Work out the finished part from the listing and answer in its coordinate system (mm). A direction names the side the tool comes from. Coordinates: 2 decimals unless noted, no trailing zeros. Order: outer loops, then holes, each group sorted by start corner. A loop starts at its lowest first (then second) coordinate and runs counter-clockwise, first axis right, second up.
1. The part is cut by section D-D, the plane y = 23.5. Give the vertices of the cut face in (x, z).
2. The part is cut by section C-C, the plane z = 4.5. Give the vertices of the cut face in (x, y), then the cut area to 3 significant figures.
3. A tool of negligible diameter and unlimited length cuts with its end or side. For faces 4 (the flat face through (0, 2, 2)), 5 (the flat face through (18, 34, 3.5)), 6 (the flat face through (18, 33, 4)), from which of +Z, -Z, +X, -X, +Y, -Y can it reach the whole face along a straight path? Write none if from no direction.
4. A flat-ended cylindrical pin translates along its axis: pin 1 Ø1.5 at (y, z) = (17, 2) entering from -X. Find the tip coordinate at first contact, or state that the pin passes through.
5. Determine the mould class of faces 1 (the flat face through (20, 0, 2)), 2 (the flat face through (18, 5, 1)), 3 (the flat face through (20, 38, 2)) for opening direction Y: +Y half, -Y half, draft (parallel to the pull), parting line (faces both ways), or undercut.
6. The part is cut by section A-A, the plane x = 19. Give the vertices of the cut face in (y, z).
7. The part is cut by section B-B, the plane y = 34. Give the vertices of the cut face in (x, z).
8. Find the intervals of material crossed by probe 1 along Y at (x, z) = (2.5, 4.85); probe 2 along Y at (x, z) = (6.5, 2.65); probe 3 along Z at (x, y) = (31, 34), in increasing order.
```python
from build123d import *

# Parameters (mm, degrees)
ESQUISSE1_W             = 41
ESQUISSE1_H             = 38
BOSS_EXTRU_1_DEPTH      = 5
ESQUISSE6_W             = 36
ESQUISSE6_H             = 21
ENL_V_MAT_EXTRU_3_DEPTH = 5
ESQUISSE7_W             = 2
ESQUISSE7_H             = 32
ENL_V_MAT_EXTRU_4_DEPTH = 36
ESQUISSE8_W             = 5
ESQUISSE8_H             = 28
ENL_V_MAT_EXTRU_5_DEPTH = 36


with BuildPart() as part:
    # Esquisse1 → Boss.-Extru.1 (new body)
    with BuildSketch(Plane.XY):
        with Locations((20.5, 19)):
            Rectangle(ESQUISSE1_W, ESQUISSE1_H)
    extrude(amount=BOSS_EXTRU_1_DEPTH)

    # Esquisse6 → Enlèv. mat.-Extru.3 (cut)
    with BuildSketch(Plane(origin=(0, 0, 0), x_dir=(-1, 0, 0), z_dir=(0, 0, -1))):
        with Locations((-18, 19)):
            Rectangle(ESQUISSE6_W, ESQUISSE6_H)
    extrude(amount=-ENL_V_MAT_EXTRU_3_DEPTH, mode=Mode.SUBTRACT)

    # Esquisse7 → Enlèv. mat.-Extru.4 (cut)
    with BuildSketch(Plane.ZY):
        with Locations((2.5, 19)):
            Rectangle(ESQUISSE7_W, ESQUISSE7_H)
    extrude(amount=-ENL_V_MAT_EXTRU_4_DEPTH, mode=Mode.SUBTRACT)

    # Esquisse8 → Enlèv. mat.-Extru.5 (cut)
    with BuildSketch(Plane.ZY):
        with Locations((2.5, 19)):
            Rectangle(ESQUISSE8_W, ESQUISSE8_H)
    extrude(amount=-ENL_V_MAT_EXTRU_5_DEPTH, mode=Mode.SUBTRACT)


solid = part.part
```
Geometry says:
1. outline: (36, 0) - (41, 0) - (41, 5) - (36, 5) - close
2. outline: (0, 0) - (41, 0) - (41, 38) - (0, 38) - (0, 33) - (36, 33) - (36, 5) - (0, 5) - close
2. area: 550 mm2
3. face 4: +Z, -Z, -X, +Y, -Y
3. face 5: -X
3. face 6: +Z, -Z, -X
4. pin 1: stops at x = 36
5. face 1: -Y half
5. face 2: undercut
5. face 3: +Y half
6. outline: (0, 0) - (5, 0) - (5, 1.5) - (3, 1.5) - (3, 3.5) - (5, 3.5) - (5, 5) - (0, 5) - close; (33, 0) - (38, 0) - (38, 5) - (33, 5) - (33, 3.5) - (35, 3.5) - (35, 1.5) - (33, 1.5) - close
7. outline: (0, 0) - (41, 0) - (41, 5) - (0, 5) - (0, 3.5) - (36, 3.5) - (36, 1.5) - (0, 1.5) - close
8. probe 1: y = 0 to 5, 33 to 38
8. probe 2: y = 0 to 3, 35 to 38
8. probe 3: z = 0 to 1.5, 3.5 to 5
